The model under review builds one solid part; all positions refer to its coordinate system, in mm. Face numbers are marked on the shaded views. A direction names the side the tool comes from. Round coordinates to 2 decimals unless told otherwise and drop trailing zeros. Order: outer loops, then holes, each group sorted by start corner. A loop starts at its lowest first (then second) coordinate and runs counter-clockwise, first axis right, second up.
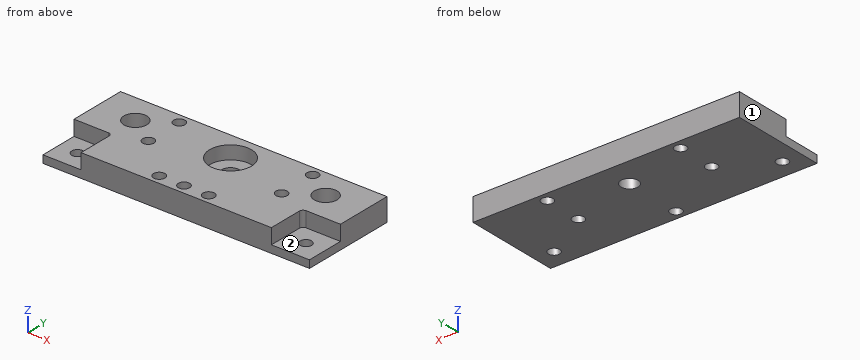
```python
from build123d import *

# Parameters (mm, degrees)
ESQUISSE1_W             = 140
ESQUISSE1_H             = 30
ESQUISSE1_R             = 11
ESQUISSE1_R_2           = 6
ESQUISSE1_R_3           = 3
EXTRUSION1_DEPTH        = 8
ESQUISSE2_W             = 140
ESQUISSE2_H             = 50
BOSS_EXTRU_1_DEPTH      = 4
ESQUISSE3_R             = 3
ENL_V_MAT_EXTRU_1_DEPTH = 5
ESQUISSE4_R             = 11
ESQUISSE4_R_2           = 3
ENL_V_MAT_EXTRU_2_DEPTH = 5
ESQUISSE5_W             = 100
ESQUISSE5_H             = 20
BOSS_EXTRU_2_DEPTH      = 8
ESQUISSE6_R             = 3
ENL_V_MAT_EXTRU_3_DEPTH = 8
ESQUISSE7_R             = 11
BOSS_EXTRU_3_DEPTH      = 5
ESQUISSE8_R             = 4.5
ENL_V_MAT_EXTRU_4_DEPTH = 6
ESQUISSE9_R             = 6
ENL_V_MAT_EXTRU_5_DEPTH = 2
ESQUISSE10_R            = 3
ENL_V_MAT_EXTRU_6_DEPTH = 13
CONG_1_R                = 2
CONG_2_R                = 2


with BuildPart() as part:
    # Esquisse1 → Extrusion1 (new body)
    with BuildSketch(Plane.XY):
        with Locations((49.95634141, -28.081325038)):
            Rectangle(ESQUISSE1_W, ESQUISSE1_H)
        with Locations((49.95634141, -28.081325038)):
            Circle(ESQUISSE1_R, mode=Mode.SUBTRACT)
        with Locations((-0.04365859, -28.081325038)):
            Circle(ESQUISSE1_R_2, mode=Mode.SUBTRACT)
        with Locations((99.95634141, -28.081325038)):
            Circle(ESQUISSE1_R_2, mode=Mode.SUBTRACT)
        with Locations((14.95634141, -18.081325038)):
            Circle(ESQUISSE1_R_3, mode=Mode.SUBTRACT)
        with Locations((14.95634141, -38.081325038)):
            Circle(ESQUISSE1_R_3, mode=Mode.SUBTRACT)
        with Locations((84.95634141, -18.081325038)):
            Circle(ESQUISSE1_R_3, mode=Mode.SUBTRACT)
        with Locations((84.95634141, -38.081325038)):
            Circle(ESQUISSE1_R_3, mode=Mode.SUBTRACT)
    extrude(amount=EXTRUSION1_DEPTH)

    # Esquisse2 → Boss.-Extru.1 (add)
    with BuildSketch(Plane(origin=(0, 0, 0), x_dir=(-1, 0, 0), z_dir=(0, 0, -1))):
        with Locations((-49.95634141, -38.081325038)):
            Rectangle(ESQUISSE2_W, ESQUISSE2_H)
    extrude(amount=BOSS_EXTRU_1_DEPTH)

    # Esquisse3 → Enlèv. mat.-Extru.1 (cut, through all)
    with BuildSketch(Plane.XY):
        with Locations((-10.04365859, -53.081325038)):
            Circle(ESQUISSE3_R)
        with Locations((109.95634141, -53.081325038)):
            Circle(ESQUISSE3_R)
    extrude(amount=-ENL_V_MAT_EXTRU_1_DEPTH, mode=Mode.SUBTRACT)

    # Esquisse4 → Enlèv. mat.-Extru.2 (cut, through all)
    with BuildSketch(Plane.XY):
        with Locations((49.95634141, -28.081325038)):
            Circle(ESQUISSE4_R)
        with Locations((14.95634141, -18.081325038)):
            Circle(ESQUISSE4_R_2)
        with Locations((14.95634141, -38.081325038)):
            Circle(ESQUISSE4_R_2)
        with Locations((84.95634141, -18.081325038)):
            Circle(ESQUISSE4_R_2)
        with Locations((84.95634141, -38.081325038)):
            Circle(ESQUISSE4_R_2)
    extrude(amount=-ENL_V_MAT_EXTRU_2_DEPTH, mode=Mode.SUBTRACT)

    # Esquisse5 → Boss.-Extru.2 (add)
    with BuildSketch(Plane.XY):
        with Locations((49.95634141, -53.081325038)):
            Rectangle(ESQUISSE5_W, ESQUISSE5_H)
    extrude(amount=BOSS_EXTRU_2_DEPTH)

    # Esquisse6 → Enlèv. mat.-Extru.3 (cut)
    with BuildSketch(Plane.XY.offset(8)):
        with Locations((62.95634141, -58.081325038)):
            Circle(ESQUISSE6_R)
        with Locations((36.95634141, -58.081325038)):
            Circle(ESQUISSE6_R)
    extrude(amount=-ENL_V_MAT_EXTRU_3_DEPTH, mode=Mode.SUBTRACT)

    # Esquisse7 → Boss.-Extru.3 (add)
    with BuildSketch(Plane(origin=(0, 0, -4), x_dir=(-1, 0, 0), z_dir=(0, 0, -1))):
        with Locations((-49.95634141, -28.081325038)):
            Circle(ESQUISSE7_R)
    extrude(amount=-BOSS_EXTRU_3_DEPTH)

    # Esquisse8 → Enlèv. mat.-Extru.4 (cut, through all)
    with BuildSketch(Plane.XY.offset(1)):
        with Locations((49.95634141, -28.081325038)):
            Circle(ESQUISSE8_R)
    extrude(amount=-ENL_V_MAT_EXTRU_4_DEPTH, mode=Mode.SUBTRACT)

    # Esquisse9 → Enlèv. mat.-Extru.5 (cut)
    with BuildSketch(Plane.XY):
        with Locations((-0.04365859, -28.081325038)):
            Circle(ESQUISSE9_R)
        with Locations((99.95634141, -28.081325038)):
            Circle(ESQUISSE9_R)
    extrude(amount=-ENL_V_MAT_EXTRU_5_DEPTH, mode=Mode.SUBTRACT)

    # Esquisse10 → Enlèv. mat.-Extru.6 (cut, through all)
    with BuildSketch(Plane.XY.offset(8)):
        with Locations((49.95634141, -58.081325038)):
            Circle(ESQUISSE10_R)
    extrude(amount=-ENL_V_MAT_EXTRU_6_DEPTH, mode=Mode.SUBTRACT)

    # Congé1
    cong_1_edges = [part.edges().sort_by_distance(p)[0] for p in [
        (-0.04365859, -43.081325038, 4),
    ]]
    fillet(cong_1_edges, radius=CONG_1_R)

    # Congé2
    cong_2_edges = [part.edges().sort_by_distance(p)[0] for p in [
        (99.95634141, -43.081325038, 4),
    ]]
    fillet(cong_2_edges, radius=CONG_2_R)


solid = part.part
```
(1) For the marked faces 1 and 2, list the 3-axis set-ups (+Z, -Z, +X, -X, +Y, -Y) from which the entire face can be reached by the end or side of a thin tool; tool diameter is ignored.
Data:
face 1: +Z, -Z, -X, +Y, -Y
face 2: +Z, +X, -Y
(2) Consider section B-B (y = -26.5). Write out the cut boundary in (x, z).
Data:
outline: (-20.04, -4) - (45.74, -4) - (45.74, 1) - (39.07, 1) - (39.07, 8) - (5.74, 8) - (5.74, -2) - (-5.83, -2) - (-5.83, 8) - (-20.04, 8) - close; (54.17, -4) - (119.96, -4) - (119.96, 8) - (105.74, 8) - (105.74, -2) - (94.17, -2) - (94.17, 8) - (60.84, 8) - (60.84, 1) - (54.17, 1) - close
(3) To check wall thickness, follow probe 1 along X at (y, z) = (-57.5, 5.25); probe 2 along X at (y, z) = (-58.5, -1.75); probe 3 along X at (y, z) = (-57, 3.5). State the ranges of each line that lie inside material, in increasing order.
Data:
probe 1: x = -0.04 to 34.01, 39.9 to 47.01, 52.9 to 60.01, 65.9 to 99.96
probe 2: x = -20.04 to 46.99, 52.93 to 119.96
probe 3: x = -0.04 to 34.16, 39.75 to 47.16, 52.75 to 60.16, 65.75 to 99.96
(4) Insertion check: pin 1 (4 mm diameter, centred on x = -12, z = 3.5, fed in from -Y); pin 2 (3.5 mm diameter, centred on x = 0, y = -27, fed in from +Z); pin 3 (6.5 mm diameter, centred on x = 50.5, y = -25, fed in from +Z); pin 4 (7 mm diameter, centred on x = 36.96, y = -58.08, fed in from +Z). Each pin has a flat end and moves straight along its axis. Give the tip position at first contact, or say it passes through.
Data:
pin 1: stops at y = -43.08
pin 2: stops at z = -2
pin 3: stops at z = 1
pin 4: stops at z = 8
(5) Consider section D-D (x = 41.5). Write out the cut boundary in (y, z).
Data:
outline: (-63.08, -4) - (-13.08, -4) - (-13.08, 8) - (-21.05, 8) - (-21.05, 1) - (-35.12, 1) - (-35.12, 8) - (-63.08, 8) - close
(6) Consider section A-A (x = -9.5). Write out the cut boundary in (y, z).
Data:
outline: (-63.08, -4) - (-56.03, -4) - (-56.03, 0) - (-63.08, 0) - close; (-50.13, -4) - (-13.08, -4) - (-13.08, 8) - (-43.08, 8) - (-43.08, 0) - (-50.13, 0) - close
(7) Consider section C-C (z = 5.5). State how many separate pieces and enclosed holes the cut face has, and give its area (3 significant figures).
Data:
separate pieces: 1
enclosed holes: 10
area: 5,400 mm2
